```python
from build123d import *

# Parameters (mm, degrees)
BOSS_EXTRUDE1_DEPTH                     = 1.5
SKETCH2_R                               = 1.6
MOT_MNT_SCREW_HOLE_DEPTH                = 34.354609876
MOT_MNT_SCREW_HOLES_COUNT               = 2
MOT_MNT_SCREW_HOLES_ANGLE               = 60
MOT_MNT_SCREW_HOLES_THE_OTHER_WAY_COUNT = 2
MOT_MNT_SCREW_HOLES_THE_OTHER_WAY_ANGLE = 60
SKETCH3_W                               = 19.8
SKETCH3_H                               = 1.5
BASE_FLANGE_DEPTH                       = 60
SKETCH4_R                               = 2.25
BASE_MNT_SCREW_HOLES_DEPTH              = 77.709125924
FILLET1_R                               = 5
CONVERT_SOLID2_START                    = -19.8
CONVERT_SOLID2_DEPTH                    = 39.6
CONVERT_SOLID2_2_DEPTH                  = 39.6


# Read off the part's stored shape, not the designer's step: Convert-Solid2
with BuildPart() as part:
    # Sketch1 → Boss-Extrude1 (new body)
    with BuildSketch(Plane.XY):
        with BuildLine():
            Line((0, 26.8), (0, 6.5))
            ThreePointArc((0, 6.5), (-6.5, 0), (0, -6.5))
            Line((0, -6.5), (0, -18.2))
            Line((0, -18.2), (-19.8, -18.2))
            Line((-19.8, -18.2), (-19.8, 7))
            ThreePointArc((-19.8, 7), (-14.000714267, 21.000714267), (0, 26.8))
        make_face()
    extrude(amount=BOSS_EXTRUDE1_DEPTH)

    # Sketch2 → mot mnt screw hole (cut, through all)
    with BuildSketch(Plane.XY.offset(1.5)):
        with Locations((-15.5, 7)):
            Circle(SKETCH2_R)
    mot_mnt_screw_hole = extrude(amount=-MOT_MNT_SCREW_HOLE_DEPTH, mode=Mode.SUBTRACT)

    # mot mnt screw holes: mot mnt screw hole ×2 about axis
    mot_mnt_screw_holes_axis = Axis((0, 7, 1.5), (0, 0, -1))
    for i in range(1, MOT_MNT_SCREW_HOLES_COUNT):
        add(mot_mnt_screw_hole.rotate(mot_mnt_screw_holes_axis, i * MOT_MNT_SCREW_HOLES_ANGLE / (MOT_MNT_SCREW_HOLES_COUNT - 1)), mode=Mode.SUBTRACT)

    # mot mnt screw holes the other way: mot mnt screw hole ×2 about axis
    mot_mnt_screw_holes_the_other_way_axis = Axis((0, 7, 1.5), (0, 0, 1))
    for i in range(1, MOT_MNT_SCREW_HOLES_THE_OTHER_WAY_COUNT):
        add(mot_mnt_screw_hole.rotate(mot_mnt_screw_holes_the_other_way_axis, i * MOT_MNT_SCREW_HOLES_THE_OTHER_WAY_ANGLE / (MOT_MNT_SCREW_HOLES_THE_OTHER_WAY_COUNT - 1)), mode=Mode.SUBTRACT)

    # Sketch3 → base flange (add)
    with BuildSketch(Plane(origin=(0, 0, 0), x_dir=(-1, 0, 0), z_dir=(0, 0, -1))):
        with Locations((9.9, -17.45)):
            Rectangle(SKETCH3_W, SKETCH3_H)
    extrude(amount=BASE_FLANGE_DEPTH)

    # Sketch4 → base mnt screw holes (cut, through all)
    with BuildSketch(Plane(origin=(0, -16.7, 0), x_dir=(1, 0, 0), z_dir=(0, 1, 0))):
        with Locations(Location((-12.5, 10, 0), (0, 0, 270))):
            Circle(SKETCH4_R)
        with Locations(Location((-12.5, 45, 0), (0, 0, 270))):
            Circle(SKETCH4_R)
    extrude(amount=-BASE_MNT_SCREW_HOLES_DEPTH, mode=Mode.SUBTRACT)

    # Fillet1
    fillet1_edges = [part.edges().sort_by_distance(p)[0] for p in [
        (-19.8, -17.45, -60),
    ]]
    fillet(fillet1_edges, radius=FILLET1_R)

    # Mirror1: part across plane


with BuildPart() as part_1:
    add(part.part)
    add(part.part.mirror(Plane(origin=(0, 0, 0), x_dir=(0, 0, 1), z_dir=(1, 0, 0))))

    # Convert-Solid2 outline → Convert-Solid2 (cut)
    with BuildSketch(Plane.YZ.offset(CONVERT_SOLID2_START)):
        with BuildLine():
            ThreePointArc((-18.2, -3), (-16.881980515, 0.181980515), (-13.7, 1.5))
            Line((-13.7, 1.5), (-18.2, 1.5))
            Line((-18.2, 1.5), (-18.2, -3))
        make_face()
    extrude(amount=CONVERT_SOLID2_DEPTH, mode=Mode.SUBTRACT)

    # Convert-Solid2 2 outline → Convert-Solid2 2 (add)
    with BuildSketch(Plane.YZ.offset(CONVERT_SOLID2_START)):
        with BuildLine():
            ThreePointArc((-16.7, -3), (-15.821320344, -0.878679656), (-13.7, 0))
            Line((-13.7, 0), (-16.7, 0))
            Line((-16.7, 0), (-16.7, -3))
        make_face()
    extrude(amount=CONVERT_SOLID2_2_DEPTH)


solid = part_1.part
```
The listing builds one solid part. Answer for the finished solid, in the listing's coordinates (mm). A direction names the side the tool comes from. Give positions to 0.01 mm unless a question says otherwise; leave off trailing zeros. Loops run counter-clockwise (first coordinate to the right, second up) from the corner with the lowest first, then second, coordinate; pieces in that order, holes last. Notation, with made-up numbers: (69, 68.25) - (85, 68.25) arc R13 cw to (85, 85.25) - close; hole circle Ø10 at (16, 16). An arc over 180 degrees is marked (long way). Return JSON: item names as keys, results as strings. Group by question number.
1. Which of the six approach directions +Z, -Z, +X, -X, +Y, -Y give full straight-line access (tool end or side, diameter ignored) to faces 5 (the cylindrical face through (-8.61, 19.074, 0.76)), 6 (the flat face through (0, 7, 0))?
2. Find section A-A (y = 0). Write down the section's boundary in (x, z), then the cut area to 3 significant figures.
3. Determine the mould class of faces 1 (the cylindrical face through (-7.403, -4.861, 0.76)), 2 (the cylindrical face through (-12.401, -17.44, -47.248)), 3 (the flat face through (0, -18.2, -31)), 4 (the flat face through (-19.8, -17, -18)) for opening direction X: pulls with the +X half, pulls with the -X half, needs draft (parallel to the pull), parting line crosses it, or undercut.
4. Given pin 1 Ø12 at (x, y) = (-14, 19) entering from -Z; pin 2 Ø3 at (x, z) = (11, -37) entering from +Y, each flat-ended and moving along its own axis, determine where each tip first touches the part or whether it passes through.
5. Find section C-C (y = 20). Write down the section's boundary in (x, z), then the cut area to 3 significant figures.
6. Find section D-D (x = 15.5). Write down the section's boundary in (y, z).
7. Find section B-B (z = -45). Write down the section's boundary in (x, y).
8. Straight lines are drawn through the part: line 1 (X direction, y = -17.75, z = -10); line 2 (Y direction, x = 4, z = -44.5); line 3 (Z direction, x = 12, y = -17). For each, find the intervals that lie inside material, in ascending order. Write a range as [from, to].
Verdict:
{
 "1": {"face 5": "+Z, -Z", "face 6": "-Z, +X, -X, +Y"},
 "2": {"outline": "(-19.8, 0) - (-6.5, 0) - (-6.5, 1.5) - (-19.8, 1.5) - close; (6.5, 0) - (19.8, 0) - (19.8, 1.5) - (6.5, 1.5) - close", "area": "39.9 mm^2"},
 "3": {"face 1": "undercut", "face 2": "undercut", "face 3": "needs draft", "face 4": "pulls with the -X half"},
 "4": {"pin 1": "stops at z = 0", "pin 2": "stops at y = -16.7"},
 "5": {"outline": "(-14.93, 0) - (-9.29, 0) - (-9.29, 1.5) - (-14.93, 1.5) - close; (-6.21, 0) - (6.21, 0) - (6.21, 1.5) - (-6.21, 1.5) - close; (9.29, 0) - (14.93, 0) - (14.93, 1.5) - (9.29, 1.5) - close", "area": "35.5 mm^2"},
 "6": {"outline": "(-18.2, -59.95) - (-16.7, -59.95) - (-16.7, -3) arc R3 cw to (-13.7, 0) - (5.4, 0) - (5.4, 1.5) - (-13.7, 1.5) arc R4.5 ccw to (-18.2, -3) - close; (8.6, 0) - (19.32, 0) - (19.32, 1.5) - (8.6, 1.5) - close"},
 "7": {"outline": "(-19.8, -18.2) - (-14.75, -18.2) - (-14.75, -16.7) - (-19.8, -16.7) - close; (-10.25, -18.2) - (10.25, -18.2) - (10.25, -16.7) - (-10.25, -16.7) - close; (14.75, -18.2) - (19.8, -18.2) - (19.8, -16.7) - (14.75, -16.7) - close"},
 "8": {"line 1": "x = [-19.8, -14.75], [-10.25, 10.25], [14.75, 19.8]", "line 2": "y = [-18.2, -16.7]", "line 3": "z = [-60, -47.19], [-42.81, -12.19], [-7.81, 0.06]"}
}
